For this review, take the finished solid that the model builds, in its own axes (mm). Coordinates: 2 decimals unless noted, no trailing zeros. Write each loop counter-clockwise with the first axis right and the second up, starting at its lowest first coordinate (ties: lowest second). Pieces come first, ordered by that corner, then holes. Notation, with made-up numbers: (-36.75, 18.25) -> (12.25, 18.25) arc R23 ccw to (12.25, 45.25) -> close; hole circle Ø2 at (-35.5, 51). An arc over 180 degrees is marked (long way). Put each result on its own line as item: value. Start each with the question number.
Item 1: Consider section A-A on z = 4.5. Give the boundary of the cut face in (x, y), and give its area (4 significant figures).
Item 2: Consider section B-B on x = 38.5. Give the boundary of the cut face in (y, z).
Item 3: Insertion check: P1, Ø2.5, axis at y = -4, z = 2, coming from the +X side; P2, Ø4, axis at y = 106, z = 4.5, coming from the -X side; P3, Ø4, axis at y = 27, z = 2.5, coming from the +X side; P4, Ø6, axis at x = 27.5, y = 77, coming from the -Z side. Each pin has a flat end and moves straight along its axis. Give the tip position at first contact, or say it passes through.
Item 4: To check wall thickness, follow L1, parallel to Y at x = 42, z = 0.5; L2, parallel to Y at x = 35.5, z = 2; L3, parallel to X at y = 53, z = 7.25. State the ranges of each line that lie inside material, in increasing order.
Item 5: Consider section C-C on y = 91. Give the boundary of the cut face in (x, z).
```python
from build123d import *

# Parameters (mm, degrees)
BOSS_EXTRU_1_DEPTH = 8
ESQUISSE2_W        = 8
ESQUISSE2_H        = 20
BOSS_EXTRU_2_DEPTH = 8
ESQUISSE3_W        = 20
ESQUISSE3_H        = 8
BOSS_EXTRU_3_DEPTH = 8


with BuildPart() as part:
    # Esquisse1 → Boss.-Extru.1 (new body)
    with BuildSketch(Plane.XY):
        Polygon((0, 0), (110, 0), (0, 115), align=None)
    extrude(amount=BOSS_EXTRU_1_DEPTH)

    # Esquisse2 → Boss.-Extru.2 (add)
    with BuildSketch(Plane.XY):
        with Locations((-4, 40)):
            Rectangle(ESQUISSE2_W, ESQUISSE2_H)
        with Locations((-4, 90)):
            Rectangle(ESQUISSE2_W, ESQUISSE2_H)
    extrude(amount=BOSS_EXTRU_2_DEPTH)

    # Esquisse3 → Boss.-Extru.3 (add)
    with BuildSketch(Plane.XY):
        with Locations((40, -4)):
            Rectangle(ESQUISSE3_W, ESQUISSE3_H)
        with Locations((90, -4)):
            Rectangle(ESQUISSE3_W, ESQUISSE3_H)
    extrude(amount=BOSS_EXTRU_3_DEPTH)


solid = part.part
```
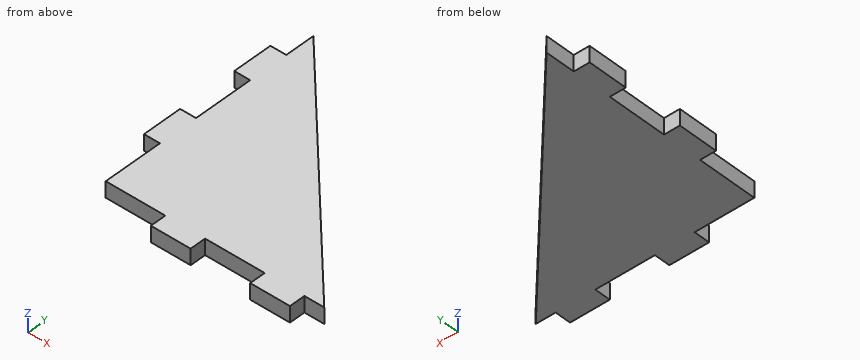
Return value:
1. outline: (-8, 30) -> (0, 30) -> (0, 0) -> (30, 0) -> (30, -8) -> (50, -8) -> (50, 0) -> (80, 0) -> (80, -8) -> (100, -8) -> (100, 0) -> (110, 0) -> (0, 115) -> (0, 100) -> (-8, 100) -> (-8, 80) -> (0, 80) -> (0, 50) -> (-8, 50) -> close
1. area: 6,965 mm^2
2. outline: (-8, 0) -> (74.75, 0) -> (74.75, 8) -> (-8, 8) -> close
3. P1: x = 100
3. P2: x = 0
3. P3: x = 86.09
3. P4: z = 0
4. L1: -8 to 71.09
4. L2: -8 to 77.89
4. L3: 0 to 59.3
5. outline: (-8, 0) -> (22.96, 0) -> (22.96, 8) -> (-8, 8) -> close
